Source: CAD feature listing. Evaluate the final solid. Frame: model axes, mm. Give positions to 0.01 mm unless a question says otherwise; leave off trailing zeros. Write each loop counter-clockwise with the first axis right and the second up, starting at its lowest first coordinate (ties: lowest second). Pieces come first, ordered by that corner, then holes. Notation, with made-up numbers: M 82.5,23.25 L 98.5,23.25 A24 cw 98.5,60.25 Z; hole C 82,54.5 d11. An arc over 180 degrees is marked long. Return JSON: item names as keys, results as strings.
Autodesk Inventor part; units mm, degrees
ref_plane "YZ Plane" through (0, 0, 0) normal (1, 0, 0) x (0, 1, 0)
ref_plane "XZ Plane" through (0, 0, 0) normal (0, 1, 0) x (-1, 0, 0)
ref_plane "XY Plane" through (0, 0, 0) normal (0, 0, 1) x (1, 0, 0)
sketch "Sketch1" plane through (0, 0, 0) normal (0, 1, 0) x (-1, 0, 0)
  line L0 (-34.333, 34.6818) -> (-49.333, 34.6818) construction
  line L1 (-34.333, -45.5191) -> (-34.333, 34.6818) construction
  line L2 (-34.333, 34.6818) -> (-49.333, -49.911) construction
  line L3 (-34.333, 34.6818) -> (-34.333, 29.6818) construction
  line L4 (-34.333, 19.6818) -> (-46.333, 19.6818) construction
  line L5 (-46.333, 19.6818) -> (-46.333, 29.6818) construction
  line L6 (-46.333, 29.6818) -> (-34.333, 29.6818) construction
  line L7 (-34.333, 3.6818) -> (-46.333, 3.6818) construction
  line L8 (-46.333, 3.6818) -> (-46.333, 13.6818) construction
  line L9 (-46.333, 13.6818) -> (-34.333, 13.6818) construction
  line L10 (-34.333, -12.3182) -> (-46.333, -12.3182) construction
  line L11 (-46.333, -12.3182) -> (-46.333, -2.3182) construction
  line L12 (-46.333, -2.3182) -> (-34.333, -2.3182) construction
  line L13 (-34.333, -28.3182) -> (-46.333, -28.3182) construction
  line L14 (-46.333, -28.3182) -> (-46.333, -18.3182) construction
  line L15 (-46.333, -18.3182) -> (-34.333, -18.3182) construction
  line L16 (-34.333, -44.3182) -> (-46.333, -44.3182) construction
  line L17 (-46.333, -44.3182) -> (-46.333, -34.3182) construction
  line L18 (-46.333, -34.3182) -> (-34.333, -34.3182) construction
  line L19 (-34.333, -60.3182) -> (-46.333, -60.3182) construction
  line L20 (-46.333, -60.3182) -> (-46.333, -50.3182) construction
  line L21 (-46.333, -50.3182) -> (-34.333, -50.3182) construction
  line L22 (-34.333, 19.6818) -> (-34.333, 13.6818) construction
  line L23 (-34.333, 3.6818) -> (-34.333, -2.3182) construction
  line L24 (-34.333, -12.3182) -> (-34.333, -18.3182) construction
  line L25 (-34.333, -28.3182) -> (-34.333, -34.3182) construction
  arc A0 (-7.5, -42.2964) -> (-7.5, 42.2964) centre (-35.5563, 0) ccw
  line L26 (-49.333, 34.6818) -> (-49.333, -65.3182) construction
  line L27 (-49.333, -65.3182) -> (-34.333, -65.3182) construction
  line L28 (-34.333, -65.3182) -> (-34.333, -60.3182) construction
  line L29 (0.7921, 54.796) -> (-7.5, 42.2964)
  line L30 (0.7921, 54.796) -> (4.9587, 52.032)
  line L31 (-1.8037, 41.8383) -> (4.9587, 52.032)
  line L32 (9.3874, 29.4913) -> (18.9468, 37.1243)
  line L33 (15.8269, 41.0315) -> (18.9468, 37.1243)
  line L34 (15.8269, 41.0315) -> (4.1052, 31.6719)
  line L35 (16.2597, 14.3103) -> (27.6972, 18.649)
  line L36 (25.9239, 23.3239) -> (27.6972, 18.649)
  line L37 (25.9239, 23.3239) -> (11.899, 18.0039)
  line L38 (18.1525, -2.2458) -> (30.3692, -1.6184)
  line L39 (30.1128, 3.375) -> (30.3692, -1.6184)
  line L40 (30.1128, 3.375) -> (15.1325, 2.6057)
  line L41 (14.8841, -18.5862) -> (26.706, -21.7303)
  line L42 (27.9911, -16.8982) -> (26.706, -21.7303)
  line L43 (27.9911, -16.8982) -> (13.495, -13.0429)
  line L44 (6.7685, -33.1405) -> (17.0595, -39.7539)
  line L45 (19.7626, -35.5476) -> (17.0595, -39.7539)
  line L46 (19.7626, -35.5476) -> (7.1437, -27.4381)
  line L47 (-5.4144, -44.51) -> (2.3568, -53.9573)
  line L48 (6.2182, -50.781) -> (2.3568, -53.9573)
  line L49 (6.2182, -50.781) -> (-3.3108, -39.1966)
  arc A1 (-5.4144, -44.51) -> (-5.8417, 44.7964) centre (-35.5563, 0) ccw
  line L50 (2.3568, -53.9573) -> (-7.329, -42.1825)
  arc A2 (0.7921, 54.796) -> (-7.5, 42.2964) centre (3.3515, 44.0979) ccw
  arc A3 (15.8269, 41.0315) -> (6.4495, 33.5438) centre (14.44, 33.1526) ccw
  arc A4 (9.3874, 29.4913) -> (18.9468, 37.1243) centre (10.9496, 37.3373) ccw
  arc A5 (25.9239, 23.3239) -> (14.704, 19.0679) centre (22.1907, 16.2484) ccw
  arc A6 (16.2597, 14.3103) -> (27.6972, 18.649) centre (20.1496, 21.301) ccw
  arc A7 (30.1128, 3.375) -> (18.1286, 2.7595) centre (24.3921, -2.2173) ccw
  arc A8 (18.1525, -2.2458) -> (30.3692, -1.6184) centre (23.9964, 3.2176) ccw
  arc A9 (27.9911, -16.8982) -> (16.3942, -13.814) centre (20.8326, -20.4699) ccw
  arc A10 (14.8841, -18.5862) -> (26.706, -21.7303) centre (22.1204, -15.1749) ccw
  arc A11 (19.7626, -35.5476) -> (9.6675, -29.06) centre (11.8543, -36.7553) ccw
  arc A12 (6.7685, -33.1405) -> (17.0595, -39.7539) centre (14.7018, -32.1092) ccw
  arc A13 (6.2182, -50.781) -> (-1.405, -41.5135) centre (-1.68, -49.5088) ccw
  arc A14 (-7.329, -42.1825) -> (2.3568, -53.9573) centre (3.6382, -43.0322) ccw
  arc A15 (-1.8037, 41.8383) -> (4.9587, 52.032) centre (-2.7195, 49.7857) ccw
  point P0 (0, 0)
  point P1 (-34.333, -5.4186)
  point P2 (-1.405, -41.5135)
  point P3 (9.6675, -29.06)
  point P4 (16.3942, -13.814)
  point P5 (18.1286, 2.7595)
  point P6 (14.704, 19.0679)
  point P7 (6.4495, 33.5438)
  point P8 (-7.5, 42.2964)
  dimension "d4" = 5
  dimension "d5" = 10
  dimension "d6" = 12
  dimension "d9" = 16
  dimension "d14" = 10
  dimension "d19" = 100
  dimension "d20" = 3
  dimension "d25" = 5
  dimension "d28" = 107
  dimension "d30" = 17.833
  dimension "d31" = 50.7557
  dimension "d32" = 11
  dimension "d34" = 8
  dimension "d35" = 8
  dimension "d36" = 8
  dimension "d37" = 8
  dimension "d38" = 8
  dimension "d39" = 8
  dimension "d40" = 8
  dimension "d41" = 8
  dimension "d42" = 8
  dimension "d43" = 8
  dimension "d44" = 8
  dimension "d46" = 11
  dimension "d47" = 8
extrude "Extrusion1" add sketch "Sketch1" along normal blind 20
properties part number "pneunet_approximate_test_first_bend_INFLATED"
1) Cut plane D-D, the plane x = -24. Return the cut outline in (y, z).
Numbers:
{"outline": "M 0,-22.95 L 20,-22.95 L 20,-13.12 L 0,-13.12 Z; M 0,-4.78 L 20,-4.78 L 20,5.77 L 0,5.77 Z; M 0,14.29 L 20,14.29 L 20,24.04 L 0,24.04 Z"}
2) Line query: line 1 (Z direction, x = -16, y = 19.25); line 2 (Z direction, x = -24, y = 9.5); line 3 (Z direction, x = -2, y = 17). Output: solid intervals per line, ascending. Write a range as [from, to].
Numbers:
{"line 1": "z = [-40, -29.91], [-20.33, 21.32], [31.13, 40.81]", "line 2": "z = [-22.95, -13.12], [-4.78, 5.77], [14.29, 24.04]", "line 3": "z = [-53.91, -42.41], [-38.46, -34.14], [34.14, 38.46], [43.33, 53.99]"}
3) Contact query for flat-ended pins moving along their axis: pin 1 Ø8 at (y, z) = (13, 38.5) entering from -X; pin 2 Ø8 at (x, y) = (3, 7) entering from +Z; pin 3 Ø3 at (y, z) = (2.5, -30.5) entering from -X; pin 4 Ø4 at (x, y) = (1.5, 15.5) entering from +Z. Output: stop coordinate, or through.
Numbers:
{"pin 1": "stops at x = -18.95", "pin 2": "stops at z = 54.8", "pin 3": "stops at x = -18.29", "pin 4": "stops at z = 54.72"}
4) Cut plane C-C, the plane y = 17. Return the cut outline in (x, z) (1 decimal), then the cut area to 3 significant figures.
Numbers:
{"outline": "M -30.4,-1.6 A8 ccw -18.2,-2.2 A53.8 ccw -16.4,-13.8 A8 ccw -28,-16.9 L -26.7,-21.7 A8 ccw -14.9,-18.6 A53.8 ccw -9.7,-29.1 A8 ccw -19.8,-35.5 L -17.1,-39.8 A8 ccw -6.8,-33.1 A53.8 ccw 1.4,-41.5 A8 ccw -6.2,-50.8 L -2.4,-54 A11 ccw 7.3,-42.2 A50.8 cw 7.5,42.3 A11 ccw -0.8,54.8 L -5,52 A8 ccw 1.8,41.8 A53.8 ccw -6.4,33.5 A8 ccw -15.8,41 L -18.9,37.1 A8 ccw -9.4,29.5 A53.8 ccw -14.7,19.1 A8 ccw -25.9,23.3 L -27.7,18.6 A8 ccw -16.3,14.3 A53.8 ccw -18.1,2.8 A8 ccw -30.1,3.4 Z", "area": "1,070 mm²"}
5) Cut plane B-B, the plane z = -38.5. Return the cut outline in (x, y), then the cut area to 3 significant figures.
Numbers:
{"outline": "M -17.87,0 L -9.89,0 L -9.89,20 L -17.87,20 Z; M -1.96,0 L 2.48,0 L 2.48,20 L -1.96,20 Z", "area": "248 mm²"}
6) Draft query along X for faces 1 (the face through (-23.887, 9.86, 5.767)), 2 (the face through (-26.798, 9.86, 21.019)), 3 (the face through (5.88, 9.86, 50.08)), 4 (the face through (-23.078, 9.86, 13.856)). Return one class per face: released by +X, released by -X, zero draft, split by the parting line, or undercut.
Numbers:
{"face 1": "undercut", "face 2": "released by -X", "face 3": "released by +X", "face 4": "undercut"}
7) Cut plane A-A, the plane x = 3.5. Return the cut outline in (y, z), then the cut area to 3 significant figures.
Numbers:
{"outline": "M 0,-51.4 L 20,-51.4 L 20,-39.35 L 0,-39.35 Z; M 0,39.35 L 20,39.35 L 20,52.7 L 0,52.7 Z", "area": "508 mm²"}
